Autodesk Inventor part; units mm, degrees
ref_plane "YZ Plane" through (0, 0, 0) normal (1, 0, 0) x (0, 1, 0)
ref_plane "XZ Plane" through (0, 0, 0) normal (0, 1, 0) x (-1, 0, 0)
ref_plane "XY Plane" through (0, 0, 0) normal (0, 0, 1) x (1, 0, 0)
sketch "Sketch1" plane through (0, 0, 0) normal (1, 0, 0) x (0, 1, 0)
  line L0 (0, -444.5) -> (444.5, 0)
  line L1 (-35.921, -408.579) -> (408.579, 35.921)
  line L2 (0, -444.5) -> (-35.921, -408.579)
  line L3 (408.579, 35.921) -> (444.5, 0)
  point P0 (0, 0)
  dimension "d1" = 444.5
  dimension "d3" = 50.8
extrude "Extrusion1" add sketch "Sketch1" along normal blind 25.4
sketch "Sketch2" plane through (0, 408.579, 35.921) normal (0, 0.7071, 0.7071) x (1, 0, 0)
  line L0 (0, 50.8) -> (0, 0)
  line L1 (0, 0) -> (25.4, 0)
  line L2 (25.4, 0) -> (25.4, 50.8)
  line L3 (25.4, 50.8) -> (0, 50.8)
  line L4 (0, 50.8) -> (0, 0)
  line L5 (3.175, 47.625) -> (22.225, 47.625)
  line L6 (22.225, 47.625) -> (22.225, 3.175)
  line L7 (22.225, 3.175) -> (3.175, 3.175)
  line L8 (3.175, 3.175) -> (3.175, 47.625)
  point P0 (0, -263.509)
  dimension "d6" = 3.175
extrude "Extrusion2" cut sketch "Sketch2" against normal blind 762 contours L5 L6 L7 L8
sketch "Sketch3" plane through (25.4, 0, 0) normal (1, 0, 0) x (0, 0, -1)
  line L0 (444.5, 0) -> (0, 444.5)
  line L1 (0, 444.5) -> (0, 339.9202)
  line L2 (0, 339.9202) -> (302.3662, 0)
  line L3 (302.3662, 0) -> (653.5481, 0)
  line L4 (653.5481, 0) -> (477.9571, -156.1918)
  line L5 (477.9571, -156.1918) -> (43.0071, -156.1918)
  line L6 (43.0071, -156.1918) -> (-176.0789, 222.25)
  line L7 (-176.0789, 222.25) -> (-134.1948, 471.4919)
  line L8 (-134.1948, 471.4919) -> (0, 494.0448)
  line L9 (0, 494.0448) -> (0, 444.5)
  point P0 (0, 0)
extrude "Extrusion3" cut sketch "Sketch3" against normal blind 25.4 contours L3 L4 L5 L6 L7 L8 L9 L1 L2
sketch "Sketch4" plane through (25.4, 0, 0) normal (1, 0, 0) x (0, 0, -1)
  line L0 (0, 0) -> (12.7, 0)
  line L1 (12.7, 0) -> (12.7, 805.7013)
  line L2 (12.7, 805.7013) -> (-196.8353, 855.7921)
  line L3 (-196.8353, 855.7921) -> (-242.5704, 324.3941)
  line L4 (-242.5704, 324.3941) -> (0, 0)
  dimension "d11" = 12.7
extrude "Extrusion4" cut sketch "Sketch4" against normal blind 25.4
properties part number "liftanglebar" material "Aluminum 6061"
Part model, mm, in its own coordinate system. A direction names the side the tool comes from. Give positions to 0.01 mm unless a question says otherwise; leave off trailing zeros. Write each loop counter-clockwise with the first axis right and the second up, starting at its lowest first coordinate (ties: lowest second). Pieces come first, ordered by that corner, then holes. Notation, with made-up numbers: (67.25, 41.5) -> (117.25, 41.5) arc R26 ccw to (117.25, 58.5) -> close; hole circle Ø10 at (66, 51.25). An arc over 180 degrees is marked (long way). Put each result on its own line as item: value. Start each with the question number.
Item 1: Cut at B-B (z = -64). List the corners of the cut face in (x, y) (3 decimals), then the cut area to 3 significant figures.
Item 2: Pin check, flat tips, straight feed: pin 1 Ø8 at (x, z) = (9.5, -182) entering from +Y; pin 2 Ø8 at (x, z) = (9.5, -209) entering from -Y; pin 3 Ø8 at (x, y) = (6.5, 226) entering from -Z. Stop position of each tip, or through.
Item 3: Which spindle directions (+Z, -Z, +X, -X, +Y, -Y) get a long thin tool onto all of the face, cutting with end or side? Do faces 4 (the face through (23, 396, -12.7)), 5 (the face through (3.175, 201, -207)). Say none if no direction does.
Item 4: Cut at C-C (y = 129). List the corners of the cut face in (x, z) (3 decimals), then the cut area to 3 significant figures.
Item 5: Cut at D-D (z = -388). List the corners of the cut face in (x, y) (3 decimals).
Item 6: Cut at A-A (x = 12.25). List the corners of the cut face in (y, z).
Item 7: Pull direction Z, two halves, no side cores. Call faces 1 (the face through (12.52, 177.46, -195.2)), 2 (the face through (12.83, 184.78, -192.37)), 3 (the face through (25.4, 199, -212)): pulls with the +Z half, pulls with the -Z half, needs draft (parallel to the pull), parting line crosses it, or undercut.
Item 8: Wall check: L1, parallel to X at y = 155, z = -274 (3 decimals); L2, parallel to Z at x = 19.5, y = 183; L3, parallel to Z at x = 15.5, y = 321. Give the ranges that are in metal, low to high. Write a range as [from, to].
Answer list:
1. outline: (0, 308.658) -> (25.4, 308.658) -> (25.4, 380.5) -> (0, 380.5) -> close; hole (3.175, 313.148) -> (22.225, 313.148) -> (22.225, 376.01) -> (3.175, 376.01) -> close
1. area: 627 mm2
2. pin 1: stops at y = 266.5
2. pin 2: stops at y = 159.66
2. pin 3: stops at z = -222.5
3. face 4: +Z, +X, -X, +Y, -Y
3. face 5: none
4. outline: (0, -315.5) -> (25.4, -315.5) -> (25.4, -243.658) -> (0, -243.658) -> close; hole (3.175, -311.01) -> (22.225, -311.01) -> (22.225, -248.148) -> (3.175, -248.148) -> close
4. area: 627 mm2
5. outline: (0, 0) -> (3.175, 0) -> (3.175, 52.01) -> (22.225, 52.01) -> (22.225, 0) -> (25.4, 0) -> (25.4, 56.5) -> (0, 56.5) -> close
6. outline: (0, -444.5) -> (431.8, -12.7) -> (427.31, -12.7) -> (0, -440.01) -> close; (0, -377.15) -> (364.45, -12.7) -> (359.96, -12.7) -> (0, -372.66) -> close
7. face 1: pulls with the +Z half
7. face 2: undercut
7. face 3: needs draft
8. L1: x = [0, 3.175], [22.225, 25.4]
8. L2: z = [-261.5, -257.01], [-194.15, -189.66]
8. L3: z = [-123.5, -119.01], [-56.15, -51.66]
